Geometry: see drawing. Coordinates: mm, zero at the bounding-box minimum. A direction names the side the tool comes from. Coordinates: 2 decimals unless noted, no trailing zeros. Order: outer loops, then holes, each group sorted by start corner. A loop starts at its lowest first (then second) coordinate and runs counter-clockwise, first axis right, second up. Notation, with made-up numbers: (-23.75, 81) - (-16.75, 81) arc R6 ccw to (-16.75, 90) - close; hole circle Ø2 at (-9.75, 4.5). An arc over 180 degrees is marked (long way). Use a Markdown table: item, result. Add a question column.
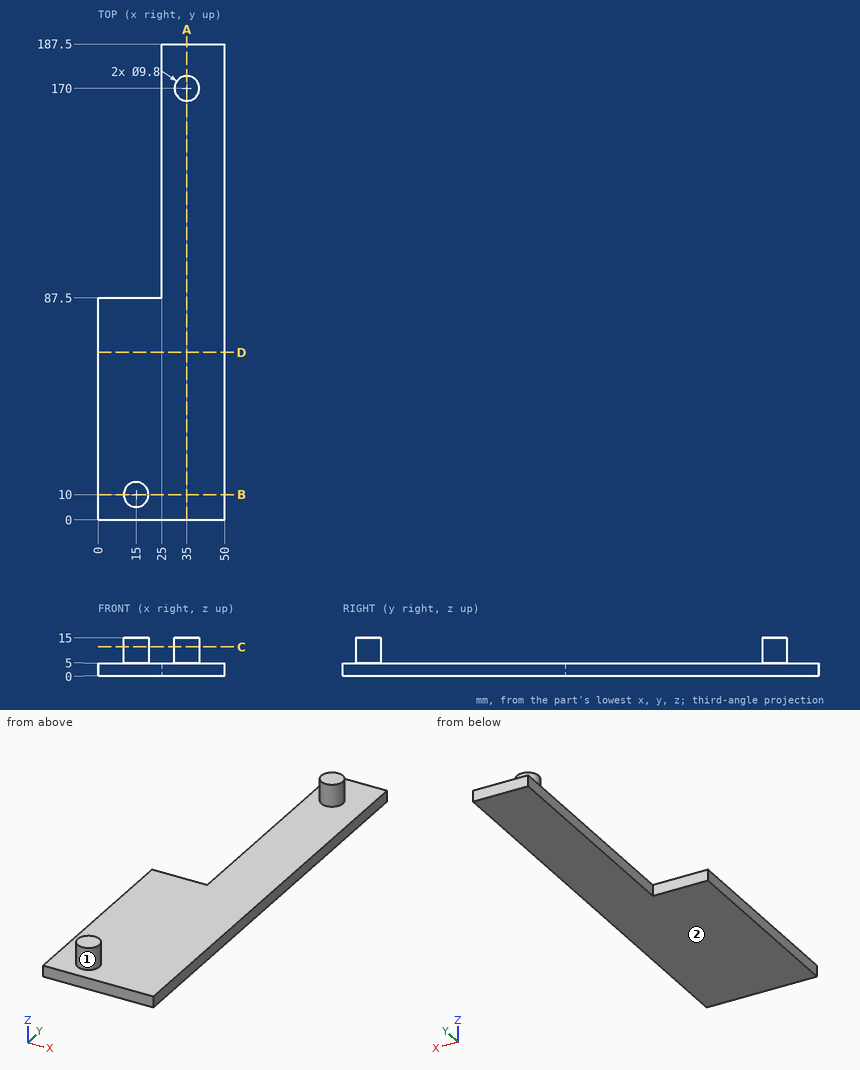
1) Cut plane A-A (x = 35). Return the cut outline in (y, z), and give its area (3 significant figures).
2) Cut plane C-C (z = 11.5). Return the cut outline in (x, y).
3) Contact query for flat-ended pins moving along their axis: P1, Ø2, axis at y = 145, z = 3.5, coming from the -X side; P2, Ø2.5, axis at x = 8.5, z = 3.5, coming from the +Y side; P3, Ø3, axis at x = 20.5, z = 9, coming from the -Y side. Output: stop coordinate, or through.
4) Cut plane B-B (y = 10). Return the cut outline in (x, z).
5) Cut plane D-D (y = 66). Return the cut outline in (x, z).
6) Reachability of the marked faces 1 and 2 from +Z, -Z, +X, -X, +Y, -Y: full face, straight path, thin tool, end or side. Return the list, or none.
7) Material intervals for L1, parallel to Y at x = 12, z = 3; L2, parallel to Z at x = 45.5, y = 165.5; L3, parallel to Y at x = 35, z = 13.75, sorted ascending.
Computed:
| question | item | result |
|---|---|---|
| 1 | outline | (0, 0) - (187.5, 0) - (187.5, 5) - (174.9, 5) - (174.9, 15) - (165.1, 15) - (165.1, 5) - (0, 5) - close |
| 1 | area | 1,040 mm2 |
| 2 | outline | circle Ø9.8 at (15, 10); circle Ø9.8 at (35, 170) |
| 3 | P1 | stops at x = 25 |
| 3 | P2 | stops at y = 87.5 |
| 3 | P3 | stops at y = 7.17 |
| 4 | outline | (0, 0) - (50, 0) - (50, 5) - (19.9, 5) - (19.9, 15) - (10.1, 15) - (10.1, 5) - (0, 5) - close |
| 5 | outline | (0, 0) - (50, 0) - (50, 5) - (0, 5) - close |
| 6 | face 1 | +Z |
| 6 | face 2 | -Z, +X, -X, +Y, -Y |
| 7 | L1 | y = 0 to 87.5 |
| 7 | L2 | z = 0 to 5 |
| 7 | L3 | y = 165.1 to 174.9 |
